Geometry check sheet. Reference: the model listing, model coordinates, mm. A direction names the side the tool comes from. Coordinates: 2 decimals unless noted, no trailing zeros. Loops run counter-clockwise (first coordinate to the right, second up) from the corner with the lowest first, then second, coordinate; pieces in that order, holes last. Notation, with made-up numbers: (-36.75, 23.25) -> (-11.75, 23.25) arc R10 ccw to (-11.75, 36.25) -> close; hole circle Ø1 at (-26, -25.75). An arc over 180 degrees is marked (long way). Answer as a JSON object with one key per item and string values.
from build123d import *

# Parameters (mm, degrees)
BOSS_EXTRUDE1_DEPTH     = 35
CUT_EXTRUDE1_DEPTH      = 1.5
CUT_EXTRUDE7_DEPTH      = 91.579854792
CUT_EXTRUDE7_DEPTH_BACK = 91.579854792
SKETCH14_R              = 1


with BuildPart() as part:
    # Sketch1 → Boss-Extrude1 (new, symmetric)
    with BuildSketch(Plane(origin=(0, 0, 0), x_dir=(1, 0, 0), z_dir=(0, 1, 0))):
        Polygon((-61.5, 0), (61.5, 0), (77.378679656, 15.878679656), (77.378679656, 31.5), (75.878679656, 31.5), (75.878679656, 16.5), (60.878679656, 1.5), (-60.878679656, 1.5), (-75.878679656, 16.5), (-75.878679656, 31.5), (-77.378679656, 31.5), (-77.378679656, 15.878679656), align=None)
    extrude(amount=BOSS_EXTRUDE1_DEPTH, both=True)

    # Sketch2 → Cut-Extrude1 (cut)
    with BuildSketch(Plane.XY):
        Polygon((0, -25), (-14.281480067, -35), (14.281480067, -35), align=None)
    extrude(amount=-CUT_EXTRUDE1_DEPTH, mode=Mode.SUBTRACT)

    # Sketch12 → Cut-Loft1 section 0
    with BuildSketch(Plane(origin=(29.689339828, 0, 29.689339828), x_dir=(-0.7071067811865465, 0, 0.7071067811865488), z_dir=(-0.7071067811865488, 0, -0.7071067811865465))):
        with BuildLine():
            Line((-44.108387387, -35), (-65.321590822, -17.200008821))
            Line((-65.321590822, -17.200008821), (-65.321590822, -35))
            Line((-65.321590822, -35), (-44.108387387, -35))
        make_face()
    # Sketch7 → Cut-Loft1 section 1
    with BuildSketch(Plane(origin=(30.75, 0, 30.75), x_dir=(0.707106781186546, 0, -0.707106781186549), z_dir=(0.707106781186549, 0, 0.707106781186546))):
        with BuildLine():
            Line((43.487067043, -35), (65.942911166, -16.157309479))
            Line((65.942911166, -16.157309479), (65.942911166, -35))
            Line((65.942911166, -35), (43.487067043, -35))
        make_face()
    cut_loft1 = loft(mode=Mode.SUBTRACT)

    # Sketch8 → Cut-Loft2 section 0
    with BuildSketch(Plane(origin=(77.378679656, 0, 0), x_dir=(0, 0, -1), z_dir=(1, 0, 0))):
        with BuildLine():
            Line((15.878679656, -16.157309479), (31.5, 2.379981476))
            Line((31.5, 2.379981476), (31.5, -35))
            Line((31.5, -35), (15.878679656, -35))
            Line((15.878679656, -35), (15.878679656, -16.157309479))
        make_face()
    # Sketch13 → Cut-Loft2 section 1
    with BuildSketch(Plane.ZY.offset(-75.878679656)):
        with BuildLine():
            Line((-31.5, 0.599982358), (-31.5, -35))
            Line((-31.5, -35), (-16.5, -35))
            Line((-16.5, -35), (-16.5, -17.200008821))
            Line((-16.5, -17.200008821), (-31.5, 0.599982358))
        make_face()
    cut_loft2 = loft(mode=Mode.SUBTRACT)

    # Mirror1: Cut-Loft1, Cut-Loft2 across plane
    add(cut_loft1.mirror(Plane(origin=(0, 0, 0), x_dir=(0, 0, 1), z_dir=(1, 0, 0))), mode=Mode.SUBTRACT)
    add(cut_loft2.mirror(Plane(origin=(0, 0, 0), x_dir=(0, 0, 1), z_dir=(1, 0, 0))), mode=Mode.SUBTRACT)

    # Sketch14 → Cut-Extrude7 (cut, two sides: drawn at the far end of the back side and taken through both)
    with BuildSketch(Plane(origin=(0, 0, 0), x_dir=(0, 0, -1), z_dir=(1, 0, 0)).offset(-CUT_EXTRUDE7_DEPTH_BACK)):
        with Locations((28.5, 26.844995369)):
            Circle(SKETCH14_R)
        with Locations((28.5, 18.689990738)):
            Circle(SKETCH14_R)
        with Locations((28.5, 10.534986107)):
            Circle(SKETCH14_R)
    extrude(amount=CUT_EXTRUDE7_DEPTH + CUT_EXTRUDE7_DEPTH_BACK, mode=Mode.SUBTRACT)


solid = part.part
1. Section check A-A, the plane y = 13.5. Record the boundary of the cut face in (x, z), then the cut area to 3 significant figures.
Evaluation:
{"outline": "(-77.38, -31.5) -> (-75.88, -31.5) -> (-75.88, -16.5) -> (-60.88, -1.5) -> (60.88, -1.5) -> (75.88, -16.5) -> (75.88, -31.5) -> (77.38, -31.5) -> (77.38, -15.88) -> (61.5, 0) -> (-61.5, 0) -> (-77.38, -15.88) -> close", "area": "295 mm^2"}
2. Mould release check, pull along X, two halves, no side actions. Record for faces 4 (the face through (-77.379, 15, -24)), 5 (the face through (69.3, 8.3, -7.8)), 6 (the face through (-75.879, 15, -24)): released by +X, released by -X, zero draft, split by the parting line, or undercut.
Evaluation:
{"face 4": "released by -X", "face 5": "released by +X", "face 6": "undercut"}
3. Tool access check on faces 1 (the face through (-69.6, 8.3, -8.1)), 2 (the face through (75.879, 15, -24)), 3 (the face through (7.24, -30.07, -0.74)). Record the directions out of +Z, -Z, +X, -X, +Y, -Y that give a thin tool (end or side, any length) a straight path to the whole face; none if there is none.
Evaluation:
{"face 1": "+Z, -X, +Y, -Y", "face 2": "-Z, +Y, -Y", "face 3": "+Z, -Z, -Y"}
4. Section check B-B, the plane x = 17.5. Record the boundary of the cut face in (y, z), then the cut area to 3 significant figures.
Evaluation:
{"outline": "(-35, -1.5) -> (35, -1.5) -> (35, 0) -> (-35, 0) -> close", "area": "105 mm^2"}
5. Thickness scan on probe 1 along Z at (x, y) = (-48.5, 11); probe 2 along X at (y, z) = (-4.5, -12.5); probe 3 along Y at (x, z) = (76.4, -28.5) (3 decimals). Record the ranges inside material, lowest first. Write a range as from..to.
Evaluation:
{"probe 1": "z = -1.5..0", "probe 2": "x = -74..-71.88, 71.88..74", "probe 3": "y = -2.341..9.535, 11.535..17.69, 19.69..25.845, 27.845..35"}
6. Depth check by flat-ended pin: P1, Ø1.8, axis at y = 10.53, z = -28.5, coming from the -X side; P2, Ø21, axis at x = -19.5, y = -15, coming from the -Z side; P3, Ø1.5, axis at x = -2, y = -16.5, coming from the +Z side; P4, Ø1.5, axis at y = -11, z = -6.5, coming from the -X side. Enter the tip coordinate at first touch or a pass-through.
Evaluation:
{"P1": "passes through", "P2": "stops at z = -1.5", "P3": "stops at z = 0", "P4": "stops at x = -68.75"}
